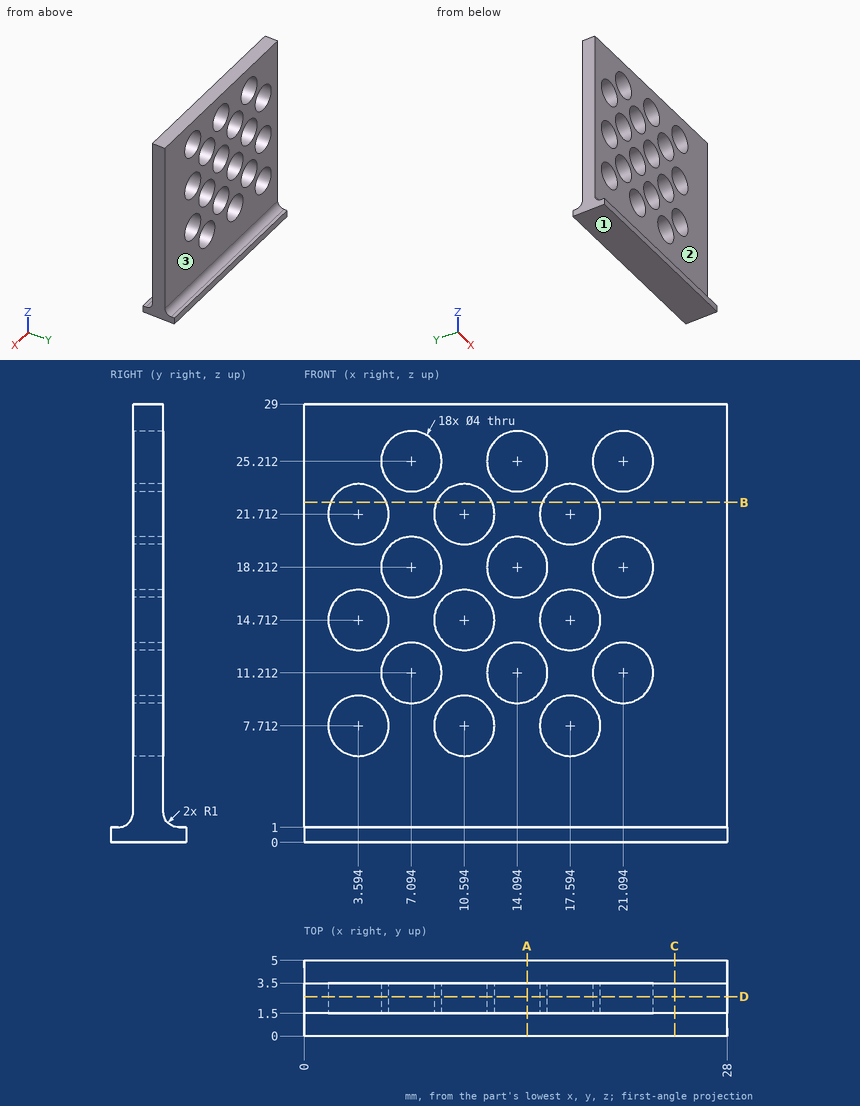
Verification items for this drawing (mm, ordinates from the low corner). A direction names the side the tool comes from. Round coordinates to 2 decimals unless told otherwise and drop trailing zeros. Loops run counter-clockwise (first coordinate to the right, second up) from the corner with the lowest first, then second, coordinate; pieces in that order, holes last. Notation, with made-up numbers: M -9.5,49.5 L 31.5,49.5 A33 cw 31.5,82.5 Z; hole C -39.5,53 d8. An arc over 180 degrees is marked long. Answer as a JSON object with one key per item and string values.
1. Access from +Z, -Z, +X, -X, +Y, -Y to the whole of each face (thin tool, end or side, straight path). Record for the marked faces 1, 2 and 3.
Reply:
{"face 1": "-Z, +X, -X, +Y, -Y", "face 2": "+Z, +X, -X, -Y", "face 3": "+Z, +X, -X, +Y"}
2. Section check C-C (x = 24.5). Record the boundary of the cut face in (y, z).
Reply:
{"outline": "M 0,0 L 5,0 L 5,1 L 4.5,1 A1 cw 3.5,2 L 3.5,29 L 1.5,29 L 1.5,2 A1 cw 0.5,1 L 0,1 Z"}
3. Gauge pin test, flat ends, axial feed: P1, Ø4.5, axis at x = 7.09, z = 18.21, coming from the -Y side; P2, Ø1.5, axis at x = 5, z = 11, coming from the +Y side. Record the tip position at first contact, or that the pin passes through.
Reply:
{"P1": "stops at y = 1.5", "P2": "stops at y = 3.5"}
4. Section check A-A (x = 14.75). Record the boundary of the cut face in (y, z).
Reply:
{"outline": "M 0,0 L 5,0 L 5,1 L 4.5,1 A1 cw 3.5,2 L 3.5,9.32 L 1.5,9.32 L 1.5,2 A1 cw 0.5,1 L 0,1 Z; M 1.5,13.1 L 3.5,13.1 L 3.5,16.32 L 1.5,16.32 Z; M 1.5,20.1 L 3.5,20.1 L 3.5,23.32 L 1.5,23.32 Z; M 1.5,27.1 L 3.5,27.1 L 3.5,29 L 1.5,29 Z"}
5. Section check B-B (z = 22.5). Record the boundary of the cut face in (x, y) (1 decimal).
Reply:
{"outline": "M 0,1.5 L 1.8,1.5 L 1.8,3.5 L 0,3.5 Z; M 5.4,1.5 L 8.8,1.5 L 8.8,3.5 L 5.4,3.5 Z; M 12.4,1.5 L 15.8,1.5 L 15.8,3.5 L 12.4,3.5 Z; M 19.4,1.5 L 28,1.5 L 28,3.5 L 19.4,3.5 Z"}
6. Section check D-D (y = 2.6). State how many separate pieces and enclosed holes the cut face has, plus the area to 3 significant figures.
Reply:
{"separate pieces": "1", "enclosed holes": "18", "area": "586 mm²"}
7. Scan lines: line 1 (Z direction, x = 17.5, y = 2.2) (1 decimal); line 2 (Z direction, x = 14.5, y = 3.3); line 3 (Y direction, x = 24.5, z = 4.25). Record each from-to range of solid material in increasing order.
Reply:
{"line 1": "z = 0 to 5.7, 9.7 to 12.7, 16.7 to 19.7, 23.7 to 29", "line 2": "z = 0 to 9.25, 13.17 to 16.25, 20.17 to 23.25, 27.17 to 29", "line 3": "y = 1.5 to 3.5"}
